Here's how the part is built. I have some questions about the finished solid (model axes, mm). A direction names the side the tool comes from. Coordinates: 2 decimals unless noted, no trailing zeros. Write each loop counter-clockwise with the first axis right and the second up, starting at its lowest first coordinate (ties: lowest second). Pieces come first, ordered by that corner, then holes.
```python
from build123d import *

# Parameters (mm, degrees)
SKETCH1_W               = 22.352
SKETCH1_H               = 15.24
SKETCH1_R               = 1.1938
BOSS_EXTRUDE1_DEPTH     = 0.8
SKETCH2_W               = 3.556
SKETCH2_H               = 5.08
BOSS_EXTRUDE2_DEPTH     = 1
CUT_EXTRUDE1_DEPTH      = 14.620843439
CUT_EXTRUDE1_DEPTH_BACK = 14.620843439
SKETCH3_R               = 0.508
SKETCH4_R               = 1.27
CUT_EXTRUDE2_DEPTH      = 0.0254


with BuildPart() as part:
    # Sketch1 → Boss-Extrude1 (new, symmetric)
    with BuildSketch(Plane(origin=(0, 0, 0), x_dir=(1, 0, 0), z_dir=(0, 1, 0))):
        Rectangle(SKETCH1_W, SKETCH1_H)
        with Locations(Location((8.636, 5.08, 0), (0, 0, 270))):
            Circle(SKETCH1_R, mode=Mode.SUBTRACT)
        with Locations(Location((8.636, -5.08, 0), (0, 0, 90))):
            Circle(SKETCH1_R, mode=Mode.SUBTRACT)
        with Locations(Location((-8.636, -5.08, 0), (0, 0, 270))):
            Circle(SKETCH1_R, mode=Mode.SUBTRACT)
        with Locations(Location((-8.636, 5.08, 0), (0, 0, 90))):
            Circle(SKETCH1_R, mode=Mode.SUBTRACT)
    extrude(amount=BOSS_EXTRUDE1_DEPTH, both=True)

    # Sketch2 → Boss-Extrude2 (add)
    with BuildSketch(Plane(origin=(0, 0.8, 0), x_dir=(1, 0, 0), z_dir=(0, 1, 0))):
        Rectangle(SKETCH2_W, SKETCH2_H)
    extrude(amount=BOSS_EXTRUDE2_DEPTH)

    # Sketch3 → Cut-Extrude1 (cut, two sides: drawn at the far end of the back side and taken through both)
    with BuildSketch(Plane(origin=(0, 0.8, 0), x_dir=(1, 0, 0), z_dir=(0, 1, 0)).offset(-CUT_EXTRUDE1_DEPTH_BACK)):
        with Locations(Location((-1.524, -5.334, 0), (0, 0, 270))):
            Circle(SKETCH3_R)
        with Locations(Location((-4.318, -5.334, 0), (0, 0, 270))):
            Circle(SKETCH3_R)
        with Locations(Location((4.318, -5.334, 0), (0, 0, 90))):
            Circle(SKETCH3_R)
        with Locations(Location((1.524, -5.334, 0), (0, 0, 90))):
            Circle(SKETCH3_R)
    extrude(amount=CUT_EXTRUDE1_DEPTH + CUT_EXTRUDE1_DEPTH_BACK, mode=Mode.SUBTRACT)

    # Sketch4 → Cut-Extrude2 (cut)
    with BuildSketch(Plane(origin=(0, 0.8, 0), x_dir=(1, 0, 0), z_dir=(0, 1, 0))):
        with Locations(Location((-4.318, -5.334, 0), (0, 0, 270))):
            Circle(SKETCH4_R)
        with Locations(Location((-1.524, -5.334, 0), (0, 0, 270))):
            Circle(SKETCH4_R)
        with Locations(Location((1.524, -5.334, 0), (0, 0, 270))):
            Circle(SKETCH4_R)
        with Locations(Location((4.318, -5.334, 0), (0, 0, 270))):
            Circle(SKETCH4_R)
    cut_extrude2 = extrude(amount=-CUT_EXTRUDE2_DEPTH, mode=Mode.SUBTRACT)

    # Mirror1: Cut-Extrude2 across plane
    add(cut_extrude2.mirror(Plane.ZX), mode=Mode.SUBTRACT)


solid = part.part
```
1) On a 3-axis mill with a long thin cutter (end or side, diameter ignored), from which of +Z, -Z, +X, -X, +Y, -Y can I reach the whole of each face in a straight line? I mean faces 1 (the face through (-2, 0.775, 6)), 2 (the face through (-2, -0.775, 6)), 3 (the face through (0, 1, -2.54)), 4 (the face through (3.89, -0.01, 5.06)), 5 (the face through (0, 1, 2.54)). Say none if no direction works.
Values follow:
face 1: +Y
face 2: -Y
face 3: -Z, +X, -X, +Y
face 4: +Y, -Y
face 5: +Z, +X, -X, +Y
2) I need wall thicknesses on probe 1 along Z at (x, y) = (8.5, -0.45); probe 2 along Z at (x, y) = (-1.5, 0.4); probe 3 along X at (y, z) = (1.5, -0.5). Which ranges of each line are inside material? Lowest first, please.
Values follow:
probe 1: z = -7.62 to -6.27, -3.89 to 3.89, 6.27 to 7.62
probe 2: z = -7.62 to 4.83, 5.84 to 7.62
probe 3: x = -1.78 to 1.78
3) Will these pins go through, and if not, where does the flat tip stop? pin 1 (1 mm diameter, centred on x = -3, z = -0.5, fed in from +Y); pin 2 (0.6 mm diameter, centred on x = -4.318, z = 5.334, fed in from -Y); pin 3 (0.8 mm diameter, centred on x = -1, z = 5, fed in from -Y); pin 4 (0.8 mm diameter, centred on y = 1.5, z = -0.5, fed in from +X).
Values follow:
pin 1: stops at y = 0.8
pin 2: passes through
pin 3: stops at y = -0.77
pin 4: stops at x = 1.78
4) Imagine slicing it at B-B on z = 0. Please give me the cut outline in (x, y), then the cut area to 3 significant figures.
Values follow:
outline: (-11.18, -0.8) - (11.18, -0.8) - (11.18, 0.8) - (1.78, 0.8) - (1.78, 1.8) - (-1.78, 1.8) - (-1.78, 0.8) - (-11.18, 0.8) - close
area: 39.3 mm2
5) Imagine slicing it at C-C on y = 0.2. Count the separate pieces of the cut face and the enclosed holes in it, then the cut area to 3 significant figures.
Values follow:
separate pieces: 1
enclosed holes: 8
area: 319 mm2
6) Imagine slicing it at A-A on z = -5.08. Please give me the cut outline in (x, y).
Values follow:
outline: (-11.18, -0.8) - (-9.83, -0.8) - (-9.83, 0.8) - (-11.18, 0.8) - close; (-7.44, -0.8) - (7.44, -0.8) - (7.44, 0.8) - (-7.44, 0.8) - close; (9.83, -0.8) - (11.18, -0.8) - (11.18, 0.8) - (9.83, 0.8) - close
7) We'd pull the mould along X, two halves only. Please class faces 6 (the face through (-3, 0.8, 0)), 7 (the face through (-1.778, 1, 0)), 8 (the face through (9.643, -0.011, -4.438)): pulls with the +X half, pulls with the -X half, needs draft (parallel to the pull), parting line crosses it, or undercut.
Values follow:
face 6: needs draft
face 7: pulls with the -X half
face 8: undercut
